Autodesk Fusion 360 part; units mm, degrees
sketch "スケッチ1" plane through (0, 0, 0) normal (0, 0, 1) x (1, 0, 0)
  line L0 (120, -17.5) -> (-120, -17.5)
  line L1 (-120, -17.5) -> (-120, 17.5)
  line L2 (-120, 17.5) -> (120, 17.5)
  line L3 (120, 17.5) -> (120, -17.5)
  line L4 (120, -17.5) -> (-120, 17.5) construction
  line L5 (-120, -17.5) -> (120, 17.5) construction
  circle A0 centre (-102, 0) radius 8
  circle A1 centre (-2, 0) radius 8
  circle A2 centre (15, 0) radius 8
  line L6 (-2, -8) -> (15, -8)
  line L7 (-2, 8) -> (15, 8)
  circle A3 centre (68, 0) radius 8
  circle A4 centre (85, 0) radius 8
  line L8 (68.0795, 7.9996) -> (84.9998, 8)
  line L9 (84.9998, -8) -> (68, -8)
  circle A5 centre (-85, 0) radius 8
  line L10 (-102, 8) -> (-85, 8)
  line L11 (-102, -8) -> (-85, -8)
  point P0 (-110, 0)
  point P1 (-102, 0)
  point P2 (-94, 0)
  point P3 (-102, 8)
  point P4 (-10, 0)
  point P5 (23, 0)
  point P6 (-2, 0)
  point P7 (15, 0)
  point P8 (60, 0)
  point P9 (68, 0)
  point P10 (85, 0)
  point P11 (93, 0)
  point P12 (-77, 0)
  point P13 (-85, 0)
  dimension "d1" = 240
  dimension "d2" = 35
  dimension "d3" = 10
  dimension "d4" = 8
  dimension "d5" = 16
  dimension "d8" = 100
  dimension "d9" = 33
  dimension "d10" = 8
  dimension "d11" = 16
  dimension "d12" = 8
  dimension "d13" = 16
  dimension "d14" = 70
  dimension "d15" = 8
  dimension "d16" = 16
  dimension "d17" = 33
  dimension "d18" = 8
  dimension "d19" = 16
  dimension "d20" = 33
  dimension "d21" = 8
  dimension "d22" = 16
  dimension "d23" = 27
extrude "押し出し1" add sketch "スケッチ1" along normal blind 6
Verification items for the finished model (mm, model axes). A direction names the side the tool comes from. Coordinates: 2 decimals unless noted, no trailing zeros. Write each loop counter-clockwise with the first axis right and the second up, starting at its lowest first coordinate (ties: lowest second). Pieces come first, ordered by that corner, then holes. Notation, with made-up numbers: M 6.5,41 L 12.5,41 A18 ccw 12.5,53 Z; hole C 10.25,18.25 d2. An arc over 180 degrees is marked long. Answer as a JSON object with one key per item and string values. Group by question number.
(1) Release check for a two-part mould opening along Y. For faces 1 (the face through (-110, 0, 3)), 2 (the face through (-2, 17.5, 3)), 3 (the face through (2, -17.5, 3)), 4 (the face through (120, 0, 3)) record: +Y half, -Y half, draft (parallel to the pull), parting line (faces both ways), or undercut.
(2) Tool access check on faces 5 (the face through (-120, 0, 3)), 6 (the face through (6, 8, 3)). Record the directions out of +Z, -Z, +X, -X, +Y, -Y that give a thin tool (end or side, any length) a straight path to the whole face; none if there is none.
(3) Cross-section at C-C, the plane x = 74. Record the cut outline in (y, z).
(4) Cross-section at B-B, the plane y = 0. Record the cut outline in (x, z).
(5) Gauge pin test, flat end, axial feed: pin 1 (1.5 mm diameter, centred on x = 87.5, y = 5, fed in from +Z). Record the tip position at first contact, or that the pin passes through.
(6) Material ranges on line 1 (X direction, y = -3.5, z = 5.5); line 2 (Y direction, x = 77.5, z = 0.4); line 3 (X direction, y = 2, z = 1), recorded low to high.
(7) Cross-section at A-A, the plane z = 2.7. Record the cut outline in (x, y), and give its area (3 significant figures).
Reply:
{
 "1": {"face 1": "undercut", "face 2": "+Y half", "face 3": "-Y half", "face 4": "draft"},
 "2": {"face 5": "+Z, -Z, -X, +Y, -Y", "face 6": "+Z, -Z"},
 "3": {"outline": "M -17.5,0 L -8,0 L -8,6 L -17.5,6 Z; M 8,0 L 17.5,0 L 17.5,6 L 8,6 Z"},
 "4": {"outline": "M -120,0 L -110,0 L -110,6 L -120,6 Z; M -77,0 L -10,0 L -10,6 L -77,6 Z; M 23,0 L 60,0 L 60,6 L 23,6 Z; M 93,0 L 120,0 L 120,6 L 93,6 Z"},
 "5": {"pin 1": "through"},
 "6": {"line 1": "-120 to -109.19, -77.81 to -9.19, 22.19 to 60.81, 92.19 to 120", "line 2": "-17.5 to -8, 8 to 17.5", "line 3": "-120 to -109.75, -77.25 to -9.75, 22.75 to 60.25, 92.75 to 120"},
 "7": {"outline": "M -120,-17.5 L 120,-17.5 L 120,17.5 L -120,17.5 Z; hole M -102,-8 L -85,-8 A8 ccw -85,8 L -102,8 A8 ccw Z; hole M -2,-8 L 15,-8 A8 ccw 15,8 L -2,8 A8 ccw Z; hole M 68,-8 L 85,-8 A8 ccw 85,8 L 68.08,8 A8 ccw long Z", "area": "6,980 mm²"}
}
